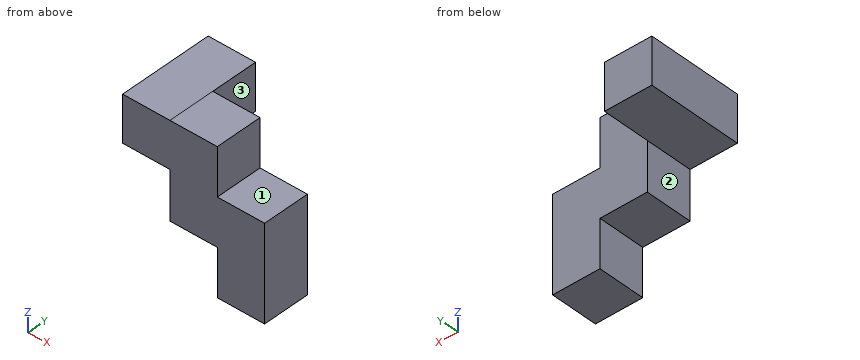
```python
from build123d import *

# Parameters (mm, degrees)
F1_DEPTH = 19.05
F2_W     = 19.05
F2_H     = 18.575629
F3_DEPTH = 19.05


with BuildPart() as f1:
    # F0 (on Front) → F1 (new body)
    with BuildSketch(Plane.XZ):
        Polygon((-34.164888, 18.575629), (-53.214888, 18.575629), (-53.214888, -19.524371), (-34.164888, -19.524371), (-34.164888, -0.474371), align=None)
        Polygon((-15.114888, -0.474371), (-34.164888, -0.474371), (-34.164888, -19.524371), (-34.164888, -38.574371), (-15.114888, -38.574371), align=None)
    extrude(amount=-F1_DEPTH)

    # F2 (on face) → F3 (join)
    with BuildSketch(Plane(origin=(-53.214888, 0, 0), x_dir=(0, -1, 0), z_dir=(-1, 0, 0))):
        with Locations((-9.525, 9.287814)):
            Rectangle(F2_W, F2_H)
        with Locations((-28.575, 9.287814)):
            Rectangle(F2_W, F2_H)
    extrude(amount=F3_DEPTH)


solid = f1.part
```
Design review of the part built by this model. Coordinates are the model's own, in mm. Face numbers are marked on the shaded views. A direction names the side the tool comes from. Give positions to 0.01 mm unless a question says otherwise; leave off trailing zeros. Order: outer loops, then holes, each group sorted by start corner. A loop starts at its lowest first (then second) coordinate and runs counter-clockwise, first axis right, second up. Notation, with made-up numbers: (-17, 48.5) - (17, 48.5) arc R26 ccw to (17, 78.5) - close; hole circle Ø10 at (87, -9.75). An arc over 180 degrees is marked (long way). Use a Markdown table: item, result. Add a question column.
(1) Add section D-D on z = -13.5. Give the boundary of the cut face in (x, y).
(2) Clearance check with flat-ended pins moving along their axes: P1, Ø5.5, axis at y = 7, z = -28.5, coming from the -X side; P2, Ø9.5, axis at x = -43.5, y = 12, coming from the -Z side; P3, Ø21, axis at x = -23, y = 13, coming from the +Z side. State where each tip first meets the part, or that it passes through.
(3) Add section C-C on x = -67. Give the boundary of the cut face in (y, z).
(4) Machinability: for the marked faces 1, 2 and 3, which of the approach directions +Z, -Z, +X, -X, +Y, -Y give a long, thin tool a straight path to every point of the face, cutting with its end or side? Answer none if there is none.
(5) Add section B-B on z = 1. Give the boundary of the cut face in (x, y), then the cut area to 3 significant figures.
(6) Wall thickness on probe 1 along Z at (x, y) = (-35, 18); probe 2 along X at (y, z) = (6.5, -5.5); probe 3 along Y at (x, z) = (-53, 0): over which ranges is each line inside the solid? List them lowest first. Write a range as [from, to].
(7) Add section A-A on y = 11. Give the boundary of the cut face in (x, z), then the cut area to 3 significant figures.
Report:
| question | item | result |
|---|---|---|
| 1 | outline | (-53.21, 0) - (-15.11, 0) - (-15.11, 19.05) - (-53.21, 19.05) - close |
| 2 | P1 | stops at x = -34.16 |
| 2 | P2 | stops at z = -19.52 |
| 2 | P3 | stops at z = -0.47 |
| 3 | outline | (0, 0) - (38.1, 0) - (38.1, 18.58) - (0, 18.58) - close |
| 4 | face 1 | +Z, +X, +Y, -Y |
| 4 | face 2 | -Z, -X, +Y, -Y |
| 4 | face 3 | +Z, -Z, +X, +Y |
| 5 | outline | (-72.26, 0) - (-34.16, 0) - (-34.16, 19.05) - (-53.21, 19.05) - (-53.21, 38.1) - (-72.26, 38.1) - close |
| 5 | area | 1,090 mm² |
| 6 | probe 1 | z = [-19.52, 18.58] |
| 6 | probe 2 | x = [-53.21, -15.11] |
| 6 | probe 3 | y = [0, 19.05] |
| 7 | outline | (-72.26, 0) - (-53.21, 0) - (-53.21, -19.52) - (-34.16, -19.52) - (-34.16, -38.57) - (-15.11, -38.57) - (-15.11, -0.47) - (-34.16, -0.47) - (-34.16, 18.58) - (-72.26, 18.58) - close |
| 7 | area | 1,810 mm² |
